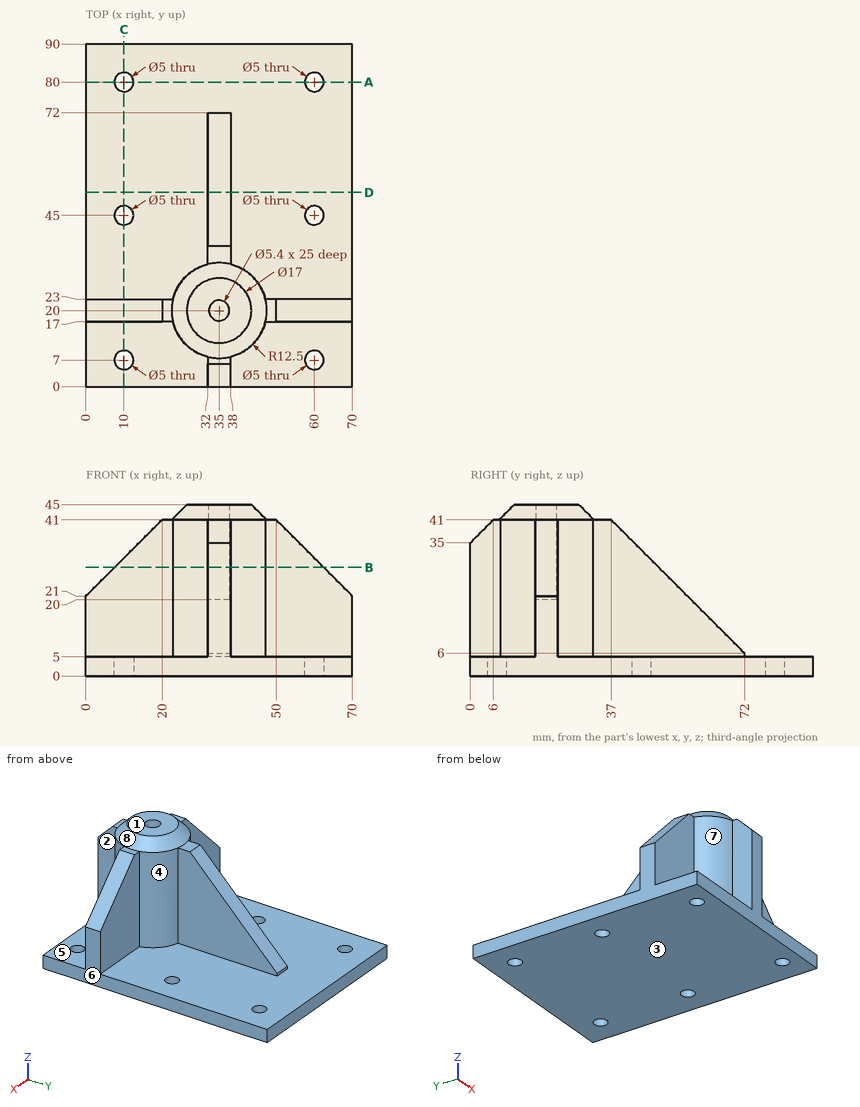
Check sheet for the drawn part. Datum: minimum x, y, z corner. Units: mm. A direction names the side the tool comes from. Coordinates: 2 decimals unless noted, no trailing zeros. Write each loop counter-clockwise with the first axis right and the second up, starting at its lowest first coordinate (ties: lowest second). Pieces come first, ordered by that corner, then holes. Notation, with made-up numbers: (-35.75, 38) - (3.25, 38) arc R18 ccw to (3.25, 66) - close; hole circle Ø11 at (55.25, -6). An arc over 180 degrees is marked (long way). Answer as a JSON object with one key per item and string values.
(1) Tool access check on the marked faces 4, 5, 6, 7 and 8. Record the directions out of +Z, -Z, +X, -X, +Y, -Y that give a thin tool (end or side, any length) a straight path to the whole face; none if there is none.
Report:
{"face 4": "+Z, +X, +Y", "face 5": "+Z, +X, -Y", "face 6": "+Z, -Z, +X, +Y, -Y", "face 7": "+Z, -X, -Y", "face 8": "+Z"}
(2) Gauge pin test, flat ends, axial feed: pin 1 Ø1 at (x, z) = (41, 17) entering from +Y (3 decimals); pin 2 Ø0.6 at (x, y) = (35.5, 7) entering from +Z; pin 3 Ø1.5 at (x, z) = (39.5, 13) entering from -Y. Record the tip position at first contact, or that the pin passes through.
Report:
{"pin 1": "y = 31.225", "pin 2": "z = 41", "pin 3": "y = 8.08"}
(3) Cross-section at D-D on y = 51. Record the cut outline in (x, z), plus the area to 3 significant figures.
Report:
{"outline": "(0, 0) - (70, 0) - (70, 5) - (38, 5) - (38, 27) - (32, 27) - (32, 5) - (0, 5) - close", "area": "482 mm^2"}
(4) Cross-section at C-C on x = 10. Record the cut outline in (y, z).
Report:
{"outline": "(0, 0) - (4.5, 0) - (4.5, 5) - (0, 5) - close; (9.5, 0) - (42.5, 0) - (42.5, 5) - (23, 5) - (23, 31) - (17, 31) - (17, 5) - (9.5, 5) - close; (47.5, 0) - (77.5, 0) - (77.5, 5) - (47.5, 5) - close; (82.5, 0) - (90, 0) - (90, 5) - (82.5, 5) - close"}
(5) Thickness scan on line 1 along Y through (x, z) = (60, 3.6); line 2 along Z through (x, y) = (28, 32); line 3 along Y through (x, z) = (19, 14). Record the ranges inside material, lowest first.
Report:
{"line 1": "0 to 4.5, 9.5 to 42.5, 47.5 to 77.5, 82.5 to 90", "line 2": "0 to 5", "line 3": "17 to 23"}
(6) Mould release check, pull along Z, two halves, no side actions. Record for the marked faces 1, 2 and 3: pulls with the +Z half, pulls with the -Z half, needs draft (parallel to the pull), parting line crosses it, or undercut.
Report:
{"face 1": "pulls with the +Z half", "face 2": "needs draft", "face 3": "pulls with the -Z half"}
(7) Cross-section at B-B on z = 28.5. Record the cut outline in (x, y).
Report:
{"outline": "(7.5, 17) - (22.87, 17) arc R12.5 ccw to (32, 7.87) - (32, 0) - (38, 0) - (38, 7.87) arc R12.5 ccw to (47.13, 17) - (62.5, 17) - (62.5, 23) - (47.13, 23) arc R12.5 ccw to (38, 32.13) - (38, 49.5) - (32, 49.5) - (32, 32.13) arc R12.5 ccw to (22.87, 23) - (7.5, 23) - close; hole circle Ø5.4 at (35, 20)"}
(8) Cross-section at A-A on y = 80. Record the cut outline in (x, z).
Report:
{"outline": "(0, 0) - (7.5, 0) - (7.5, 5) - (0, 5) - close; (12.5, 0) - (57.5, 0) - (57.5, 5) - (12.5, 5) - close; (62.5, 0) - (70, 0) - (70, 5) - (62.5, 5) - close"}
